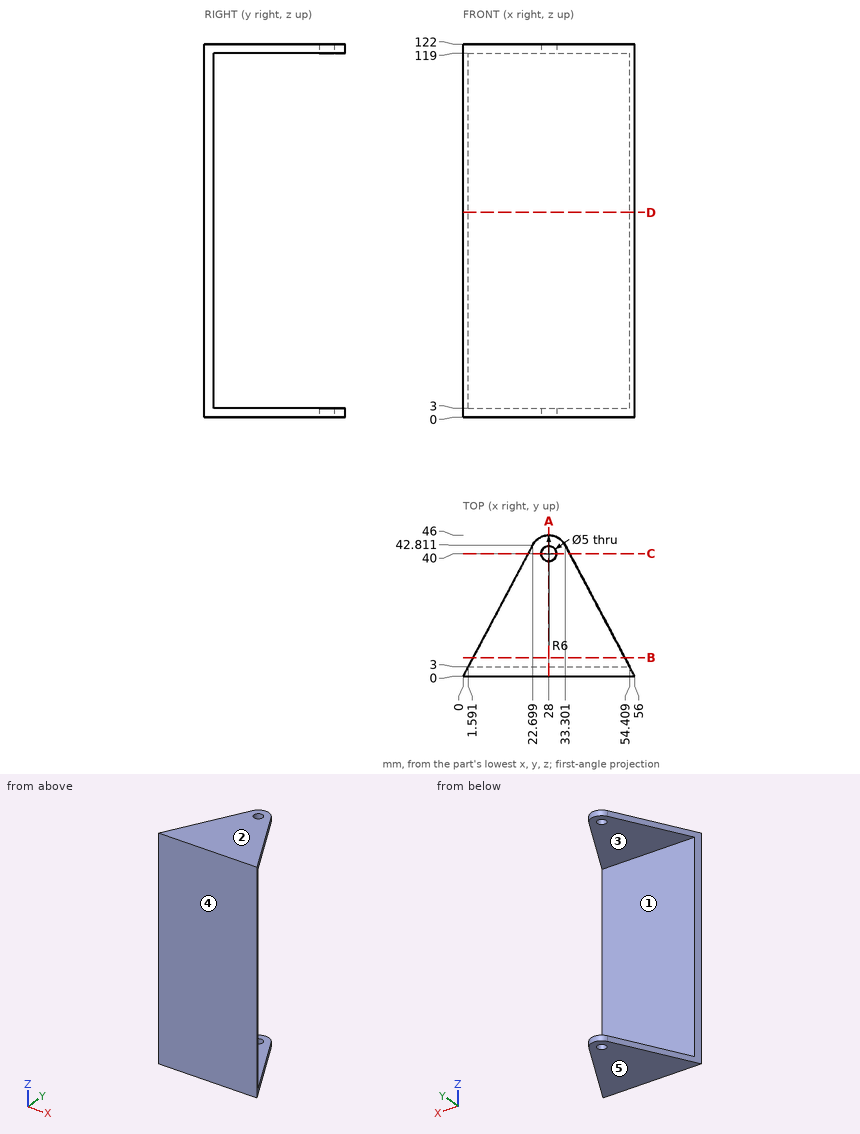
For this review, use the dimensioned drawing (mm, ordinates from the lowest corner) and the shaded views. A direction names the side the tool comes from. Round coordinates to 2 decimals unless told otherwise and drop trailing zeros. Order: outer loops, then holes, each group sorted by start corner. A loop starts at its lowest first (then second) coordinate and runs counter-clockwise, first axis right, second up. Notation, with made-up numbers: (42, -37.75) -> (87, -37.75) arc R13 ccw to (87, -12.75) -> close; hole circle Ø7 at (-22, 30). An arc over 180 degrees is marked (long way). Use CSV: the item, a comma, the result in double quotes. Start each with the question number.
(1) Consider section D-D on z = 67. Write out the cut boundary in (x, y).
(2) Consider section C-C on y = 40. Write out the cut boundary in (x, z).
(3) Insertion check: pin 1 (4 mm diameter, centred on x = 15, z = 33, fed in from +Y). The pin has a flat end and moves straight along its axis. Give the tip position at first contact, or say it passes through.
(4) Tool access review of the marked faces 1 and 2: name each direction out of +Z, -Z, +X, -X, +Y, -Y from which nothing blocks a thin tool from reaching the whole face with its end or side.
(5) Consider section B-B on y = 6. Write out the cut boundary in (x, z), and give its area (3 significant figures).
(6) Wall thickness on probe 1 along Z at (x, y) = (36, 26.5); probe 2 along Y at (x, z) = (28, 120.5); probe 3 along Y at (x, z) = (38, 26): over which ranges is each line inside the solid? List them lowest first. Write a range as from..to.
(7) Consider section A-A on x = 28. Write out the cut boundary in (y, z), and give its area (3 significant figures).
(8) Mouldability with a two-part tool opening along Z and no side actions: class the marked faces 3, 4 and 5 as pulls with the +Z half, pulls with the -Z half, needs draft (parallel to the pull), parting line crosses it, or undercut.
Responses:
1,outline,"(0, 0) -> (56, 0) -> (54.41, 3) -> (1.59, 3) -> close"
2,outline,"(21.21, 0) -> (25.5, 0) -> (25.5, 3) -> (21.21, 3) -> close; (21.21, 119) -> (25.5, 119) -> (25.5, 122) -> (21.21, 122) -> close; (30.5, 0) -> (34.79, 0) -> (34.79, 3) -> (30.5, 3) -> close; (30.5, 119) -> (34.79, 119) -> (34.79, 122) -> (30.5, 122) -> close"
3,pin 1,"y = 3"
4,face 1,"+X, -X, +Y"
4,face 2,"+Z, +X, -X, +Y, -Y"
5,outline,"(3.18, 0) -> (52.82, 0) -> (52.82, 3) -> (3.18, 3) -> close; (3.18, 119) -> (52.82, 119) -> (52.82, 122) -> (3.18, 122) -> close"
5,area,"298 mm²"
6,probe 1,"0..3, 119..122"
6,probe 2,"0..37.5, 42.5..46"
6,probe 3,"0..3"
7,outline,"(0, 0) -> (37.5, 0) -> (37.5, 3) -> (3, 3) -> (3, 119) -> (37.5, 119) -> (37.5, 122) -> (0, 122) -> close; (42.5, 0) -> (46, 0) -> (46, 3) -> (42.5, 3) -> close; (42.5, 119) -> (46, 119) -> (46, 122) -> (42.5, 122) -> close"
7,area,"594 mm²"
8,face 3,"undercut"
8,face 4,"needs draft"
8,face 5,"pulls with the -Z half"
